Source: CAD feature listing. Evaluate the final solid. Frame: model axes, mm. A direction names the side the tool comes from. Round coordinates to 2 decimals unless told otherwise and drop trailing zeros. Order: outer loops, then holes, each group sorted by start corner. A loop starts at its lowest first (then second) coordinate and runs counter-clockwise, first axis right, second up. Notation, with made-up numbers: (-23, 39) - (5, 39) arc R4 ccw to (5, 43) - close; hole circle Ø11 at (52, 50.25). An arc over 180 degrees is marked (long way). Use one line per item in the form item = value. Start each with the question number.
Q1. Ray query, line 1 (Y direction, x = 13.75, z = 6.5) (3 decimals); line 2 (Y direction, x = -10, z = 17.75) (3 decimals); line 3 (Z direction, x = 2, y = -11.75). Return the intervals inside material, ascending. Write a range as [from, to].
Q2. Cut plane A-A, the plane z = 12. Give the number of separate pieces and of enclosed holes in the cut face, and give its area (3 significant figures).
Q3. Draft query along Z for faces 1 (the flat face through (-8.01, 0.14, 23.44)), 2 (the flat face through (-6, 13.675, 14)), 3 (the flat face through (-20.15, 0, 4)), 4 (the flat face through (7.5, 0.1, 0.5)). Return one class per face: released by +Z, released by -Z, zero draft, split by the parting line, or undercut.
Q4. Pin query (flat end, axial travel): pin 1 Ø8.5 at (y, z) = (-0.5, 12.5) entering from -X; pin 2 Ø12 at (y, z) = (1.5, 16) entering from +X; pin 3 Ø2 at (x, z) = (5, 21.5) entering from -Y (3 decimals). Return the tip coordinate at first contact, or that it passes through.
Q5. Set-up query: faces 5 (the flat face through (-9, 9.875, 7)), 6 (the flat face through (19.15, 0, 14)), 7 (the cylindrical face through (0.37, -14.18, 3.51)). Return all of +Z, -Z, +X, -X, +Y, -Y with unobstructed straight access to the full face (end or side cutting, diameter ignored); none if empty.
Q6. Cut plane D-D, the plane z = 5.25. Return the cut outline in (x, y) (3 decimals).
from build123d import *

# Parameters (mm, degrees)
CROQUIS1_W              = 40.3
CROQUIS1_H              = 19.75
SALIENTE_EXTRUIR1_DEPTH = 26
CROQUIS2_W              = 14
CROQUIS2_H              = 1
CORTAR_EXTRUIR1_DEPTH   = 20
CROQUIS3_R              = 2
CORTAR_EXTRUIR2_DEPTH   = 26
CROQUIS4_R              = 9.5
SALIENTE_EXTRUIR2_DEPTH = 4.8
CROQUIS5_R              = 5
CORTAR_EXTRUIR3_DEPTH   = 30
CROQUIS6_R              = 8.5
CROQUIS6_R_2            = 5.7
CORTAR_EXTRUIR4_DEPTH   = 1
CHAFL_N1_SIZE           = 1
CHAFL_N2_SIZE           = 0.7


with BuildPart() as part:
    # Croquis1 → Saliente-Extruir1 (new body)
    with BuildSketch(Plane.XY):
        Rectangle(CROQUIS1_W, CROQUIS1_H)
    extrude(amount=SALIENTE_EXTRUIR1_DEPTH)

    # Croquis2 → Cortar-Extruir1 (cut)
    with BuildSketch(Plane(origin=(0, 9.875, 0), x_dir=(1, 0, 0), z_dir=(0, 1, 0))):
        Polygon((-19.15, -9), (-20.15, -9), (-20.15, -26), (-5.45, -26), (-10.65, -20.8), (-19.15, -20.8), align=None)
        Polygon((20.15, -26), (20.15, -9), (19.15, -9), (19.15, -20.8), (10.65, -20.8), (5.45, -26), align=None)
        with Locations((0, -0.5)):
            Rectangle(CROQUIS2_W, CROQUIS2_H)
    extrude(amount=-CORTAR_EXTRUIR1_DEPTH, mode=Mode.SUBTRACT)

    # Croquis3 → Cortar-Extruir2 (cut)
    with BuildSketch(Plane(origin=(0, 0, 0), x_dir=(-1, 0, 0), z_dir=(0, 0, -1))):
        with Locations((-13.75, 0)):
            Circle(CROQUIS3_R)
        with Locations((13.75, 0)):
            Circle(CROQUIS3_R)
    extrude(amount=-CORTAR_EXTRUIR2_DEPTH, mode=Mode.SUBTRACT)

    # Croquis4 → Saliente-Extruir2 (add)
    with BuildSketch(Plane.XZ.offset(9.875)):
        with Locations(Location((0, 12, 0), (0, 0, 90))):
            Circle(CROQUIS4_R)
    saliente_extruir2 = extrude(amount=SALIENTE_EXTRUIR2_DEPTH)

    # Simetría1: Saliente-Extruir2 across plane
    add(saliente_extruir2.mirror(Plane.ZX))

    # Croquis5 → Cortar-Extruir3 (cut)
    with BuildSketch(Plane.XZ.offset(14.675)):
        with Locations(Location((0, 12, 0), (0, 0, 270))):
            Circle(CROQUIS5_R)
    extrude(amount=-CORTAR_EXTRUIR3_DEPTH, mode=Mode.SUBTRACT)

    # Croquis6 → Cortar-Extruir4 (cut)
    with BuildSketch(Plane(origin=(0, 14.675, 0), x_dir=(1, 0, 0), z_dir=(0, 1, 0))):
        with Locations(Location((0, -12, 0), (0, 0, 270))):
            Circle(CROQUIS6_R)
        with Locations(Location((0, -12, 0), (0, 0, 270))):
            Circle(CROQUIS6_R_2, mode=Mode.SUBTRACT)
    cortar_extruir4 = extrude(amount=-CORTAR_EXTRUIR4_DEPTH, mode=Mode.SUBTRACT)

    # Simetría2: Cortar-Extruir4 across plane
    add(cortar_extruir4.mirror(Plane.ZX), mode=Mode.SUBTRACT)

    # Chaflán1
    chafl_n1_edges = [part.edges().sort_by_distance(p)[0] for p in [
        (-19.15, 0, 20.8),
        (-20.15, 0, 9),
        (19.15, 0, 20.8),
        (20.15, 0, 9),
        (-20.15, 0, 0),
        (20.15, 0, 0),
        (7, 0, 0),
        (-7, 0, 0),
    ]]
    chamfer(chafl_n1_edges, length=CHAFL_N1_SIZE - 0.0001)  # a hair under: the kernel refuses the full size

    # Chaflán2
    chafl_n2_edges = [part.edges().sort_by_distance(p)[0] for p in [
        (15.75, 0, 20.8),
        (15.75, 0, 0),
        (-11.75, 0, 20.8),
        (-11.75, 0, 0),
    ]]
    chamfer(chafl_n2_edges, length=CHAFL_N2_SIZE)


solid = part.part
Completed:
q1.line_1 = [-9.875, -2], [2, 9.875]
q1.line_2 = [-9.875, 9.875]
q1.line_3 = [2.71, 7.42], [16.58, 21.29]
q2.separate_pieces = 2
q2.enclosed_holes = 2
q2.area = 609 mm2
q3.face_1 = released by +Z
q3.face_2 = undercut
q3.face_3 = zero draft
q3.face_4 = released by -Z
q4.pin_1 = -19.9
q4.pin_2 = 19.15
q4.pin_3 = -9.875
q5.face_5 = +Y
q5.face_6 = +Z, +X, +Y, -Y
q5.face_7 = -Y
q6.outline = (-20.15, -9.875) - (-6.685, -9.875) - (-6.685, -14.675) - (-5.166, -14.675) - (-5.166, -13.675) - (5.166, -13.675) - (5.166, -14.675) - (6.685, -14.675) - (6.685, -9.875) - (20.15, -9.875) - (20.15, 9.875) - (6.685, 9.875) - (6.685, 14.675) - (5.166, 14.675) - (5.166, 13.675) - (-5.166, 13.675) - (-5.166, 14.675) - (-6.685, 14.675) - (-6.685, 9.875) - (-20.15, 9.875) - close; hole circle Ø4 at (-13.75, 0); hole circle Ø4 at (13.75, 0)
